from build123d import *

# Parameters (mm, degrees)
BOSS_EXTRUDE1_DEPTH = 6.35
SKETCH3_R           = 14.2875
SKETCH3_R_2         = 2.032
CUT_EXTRUDE1_DEPTH  = 6.35


with BuildPart() as part:
    # Sketch2 → Boss-Extrude1 (new body)
    with BuildSketch(Plane.XY):
        Polygon((-125.79203122, -159.641560721), (-74.99203122, -159.641560721), (-68.64203122, -159.641560721), (-68.64203122, -108.841560721), (-74.99203122, -108.841560721), (-74.99203122, -19.941560721), (32.95796878, -19.941560721), (32.95796878, 30.858439279), (-125.79203122, 30.858439279), (-125.79203122, -140.591560721), align=None)
    extrude(amount=BOSS_EXTRUDE1_DEPTH)

    # Sketch3 → Cut-Extrude1 (cut)
    with BuildSketch(Plane.XY.offset(6.35)):
        with Locations((-101.619115086, -20.612163927)):
            Circle(SKETCH3_R)
        with Locations((2.266884914, 10.121836073)):
            Circle(SKETCH3_R)
        with Locations((-87.69203122, -146.941560721)):
            Circle(SKETCH3_R_2)
        with Locations((-113.09203122, -146.941560721)):
            Circle(SKETCH3_R_2)
        with Locations((-100.39203122, -146.941560721)):
            Circle(SKETCH3_R_2)
        with Locations((-74.99203122, -146.941560721)):
            Circle(SKETCH3_R_2)
        with Locations((-113.09203122, -121.541560721)):
            Circle(SKETCH3_R_2)
        with Locations((-87.69203122, -121.541560721)):
            Circle(SKETCH3_R_2)
        with Locations((-74.99203122, -121.541560721)):
            Circle(SKETCH3_R_2)
        with Locations((-100.39203122, -121.541560721)):
            Circle(SKETCH3_R_2)
    extrude(amount=-CUT_EXTRUDE1_DEPTH, mode=Mode.SUBTRACT)


solid = part.part
The listing builds one solid part. Answer for the finished solid, in the listing's coordinates (mm). A direction names the side the tool comes from. Round coordinates to 2 decimals unless told otherwise and drop trailing zeros. Order: outer loops, then holes, each group sorted by start corner. A loop starts at its lowest first (then second) coordinate and runs counter-clockwise, first axis right, second up. Notation, with made-up numbers: M 8,66 L 66,66 A14 cw 66,74 Z; hole C 10,-28.5 d11. An arc over 180 degrees is marked long. Answer in a Markdown table with one row per item. Add a question column.
1) Consider line 1 along Y through (x, z) = (-114.5, 4); line 2 along X through (y, z) = (8, 6); line 3 along Y through (x, z) = (-12.5, 6.25). Determine where each line is inside the solid, lowest interval first. Write a range as from..to.
2) The part is cut by section C-C on z = 2.5. Count the separate pieces of the cut face and the enclosed holes in it, plus the area to 3 significant figures.
3) Determine the mould class of faces 4 (the face through (-98, -159.642, 3)), 5 (the face through (-112, -119.83, 3.22)), 6 (the face through (32.958, 5, 3)), 7 (the face through (-87.957, -119.527, 3.219)) for opening direction Y: pulls with the +Y half, pulls with the -Y half, needs draft (parallel to the pull), parting line crosses it, or undercut.
4) The part is cut by section D-D on y = -76. Determine the outline of the cut face in (x, z).
5) Flat-ended cylindrical pins translate along their axes: pin 1 Ø1.9 at (x, z) = (-12, 3.5) entering from -Y; pin 2 Ø3.5 at (x, y) = (-100.39, -146.94) entering from -Z; pin 3 Ø1.9 at (y, z) = (-86.5, 4.5) entering from +X; pin 4 Ø1 at (y, z) = (-128.5, 1) entering from +X. Find the tip coordinate at first contact, or state that the pin passes through.
6) The part is cut by section A-A on x = -105. Determine the outline of the cut face in (y, z), plus the area to 3 significant figures.
7) The part is cut by section B-B on y = -31.5. Determine the outline of the cut face in (x, z).
8) Which of the six approach directions +Z, -Z, +X, -X, +Y, -Y give full straight-line access (tool end or side, diameter ignored) to faces 1 (the face through (-68.642, -135, 3)), 2 (the face through (-98.454, -120.931, 3.219)), 3 (the face through (-72, -108.842, 3))?
Findings below:
| question | item | result |
|---|---|---|
| 1 | line 1 | y = -159.64..-148.41, -145.48..-123.01, -120.08..-26.79, -14.43..30.86 |
| 1 | line 2 | x = -125.79..-11.86, 16.4..32.96 |
| 1 | line 3 | y = -19.94..30.86 |
| 2 | separate pieces | 1 |
| 2 | enclosed holes | 10 |
| 2 | area | 14,100 mm² |
| 3 | face 4 | pulls with the -Y half |
| 3 | face 5 | undercut |
| 3 | face 6 | needs draft |
| 3 | face 7 | undercut |
| 4 | outline | M -125.79,0 L -74.99,0 L -74.99,6.35 L -125.79,6.35 Z |
| 5 | pin 1 | stops at y = -19.94 |
| 5 | pin 2 | passes through |
| 5 | pin 3 | stops at x = -74.99 |
| 5 | pin 4 | stops at x = -68.64 |
| 6 | outline | M -159.64,0 L -34.49,0 L -34.49,6.35 L -159.64,6.35 Z; M -6.73,0 L 30.86,0 L 30.86,6.35 L -6.73,6.35 Z |
| 6 | area | 1,030 mm² |
| 7 | outline | M -125.79,0 L -110.87,0 L -110.87,6.35 L -125.79,6.35 Z; M -92.37,0 L -74.99,0 L -74.99,6.35 L -92.37,6.35 Z |
| 8 | face 1 | +Z, -Z, +X, -Y |
| 8 | face 2 | +Z, -Z |
| 8 | face 3 | +Z, -Z, +X |
